Check sheet for the modelled part. Datum: model origin and axes. Units: mm. Face numbers are marked on the shaded views. A direction names the side the tool comes from. Give positions to 0.01 mm unless a question says otherwise; leave off trailing zeros. Order: outer loops, then holes, each group sorted by start corner. A loop starts at its lowest first (then second) coordinate and runs counter-clockwise, first axis right, second up. Notation, with made-up numbers: (65, 25.5) -> (95, 25.5) arc R21 ccw to (95, 50.5) -> close; hole circle Ø7 at (22.25, 71.5). An arc over 180 degrees is marked (long way). One line per question, with ' | ' between items.
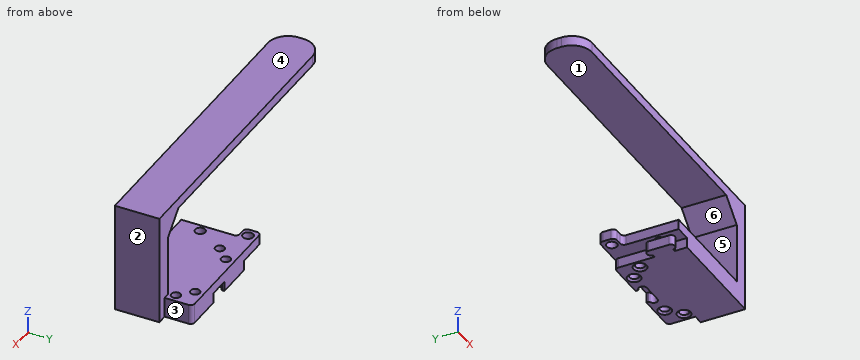
Autodesk Inventor part; units mm, degrees
ref_plane "YZ Plane" through (0, 0, 0) normal (1, 0, 0) x (0, 1, 0)
ref_plane "XZ Plane" through (0, 0, 0) normal (0, 1, 0) x (-1, 0, 0)
ref_plane "XY Plane" through (0, 0, 0) normal (0, 0, 1) x (1, 0, 0)
ref_plane "Arbeitsebene1" through (0, 0, 0) normal (0, 0, 1) x (1, 0, 0)
sketch "Skizze1" plane through (0, 0, 0) normal (0, 0, 1) x (1, 0, 0)
  circle A0 centre (-6.0705, 15.2895) radius 3.5
  circle A1 centre (15.2895, -6.0705) radius 3.5
  line L0 (30.5395, 32.5395) -> (0.0395, 32.5395)
  arc A2 (32.5395, 30.5395) -> (30.5395, 32.5395) centre (30.5395, 30.5395) ccw
  line L1 (32.5395, 30.5395) -> (32.5395, 0.0395)
  arc A3 (30.5395, -1.9605) -> (32.5395, 0.0395) centre (30.5395, 0.0395) ccw
  line L2 (0.0395, -1.9605) -> (30.5395, -1.9605)
  arc A4 (-1.9605, 0.0395) -> (0.0395, -1.9605) centre (0.0395, 0.0395) ccw
  line L3 (-1.9605, 0.0395) -> (-1.9605, 30.5395)
  arc A5 (0.0395, 32.5395) -> (-1.9605, 30.5395) centre (0.0395, 30.5395) ccw
  circle A6 centre (-4.7105, -4.7105) radius 2.45
  circle A7 centre (0.7895, -5.5105) radius 2.3
  circle A8 centre (-5.5105, 0.7895) radius 2.3
  circle A9 centre (-5.5105, 29.7895) radius 2.3
  circle A10 centre (0.7895, 36.0895) radius 2.3
  circle A11 centre (-4.7105, 35.2895) radius 2.45
  circle A12 centre (36.0895, 0.7895) radius 2.3
  circle A13 centre (29.7895, -5.5105) radius 2.3
  circle A14 centre (35.2895, -4.7105) radius 2.45
  circle A15 centre (36.0895, 29.7895) radius 2.3
  circle A16 centre (29.7895, 36.0895) radius 2.3
  circle A17 centre (35.2895, 35.2895) radius 2.45
  line L4 (20.4019, 40.2895) -> (20.4019, 39.1582)
  arc A18 (20.4019, 39.1582) -> (20.6778, 38.7524) centre (20.7437, 39.0939) ccw
  arc A19 (20.2895, 34.6895) -> (20.6778, 38.7524) centre (20.2895, 36.7395) ccw
  line L5 (20.2895, 34.6895) -> (10.1895, 34.6895)
  arc A20 (9.8548, 38.762) -> (10.1895, 34.6895) centre (10.1895, 36.7395) ccw
  arc A21 (9.8548, 38.762) -> (10.1895, 39.1567) centre (9.7895, 39.1567) ccw
  line L6 (10.1895, 39.1567) -> (10.1895, 40.2895)
  line L7 (10.1895, 40.2895) -> (-7.7105, 40.2895)
  arc A22 (-7.7105, 40.2895) -> (-9.7105, 38.2895) centre (-7.7105, 38.2895) ccw
  line L8 (-9.7105, 20.2895) -> (-9.7105, 38.2895)
  line L9 (-10.8433, 20.2895) -> (-9.7105, 20.2895)
  arc A23 (-11.3366, 20.7079) -> (-10.8433, 20.2895) centre (-10.8433, 20.7895) ccw
  arc A24 (-11.3366, 20.7079) -> (-15.2105, 20.3895) centre (-13.2605, 20.3895) ccw
  line L10 (-15.2105, 10.2895) -> (-15.2105, 20.3895)
  arc A25 (-15.2105, 10.2895) -> (-11.3515, 9.8916) centre (-13.2605, 10.2895) ccw
  arc A26 (-10.862, 10.2895) -> (-11.3515, 9.8916) centre (-10.862, 9.7895) ccw
  line L11 (-9.7105, 10.2895) -> (-10.862, 10.2895)
  line L12 (-9.7105, -7.7105) -> (-9.7105, 10.2895)
  arc A27 (-9.7105, -7.7105) -> (-7.7105, -9.7105) centre (-7.7105, -7.7105) ccw
  line L13 (-7.7105, -9.7105) -> (10.2895, -9.7105)
  line L14 (10.2895, -10.8433) -> (10.2895, -9.7105)
  arc A28 (9.8712, -11.3366) -> (10.2895, -10.8433) centre (9.7895, -10.8433) ccw
  arc A29 (9.8712, -11.3366) -> (10.1895, -15.2105) centre (10.1895, -13.2605) ccw
  line L15 (20.2895, -15.2105) -> (10.1895, -15.2105)
  arc A30 (20.2895, -15.2105) -> (20.6875, -11.3515) centre (20.2895, -13.2605) ccw
  arc A31 (20.2895, -10.862) -> (20.6875, -11.3515) centre (20.7895, -10.862) ccw
  line L16 (20.2895, -9.7105) -> (20.2895, -10.862)
  line L17 (20.2895, -9.7105) -> (38.2895, -9.7105)
  arc A32 (38.2895, -9.7105) -> (40.2895, -7.7105) centre (38.2895, -7.7105) ccw
  line L18 (40.2895, 10.1772) -> (40.2895, -7.7105)
  line L19 (40.2895, 10.1772) -> (39.1582, 10.1772)
  arc A33 (39.1582, 10.1772) -> (38.7524, 9.9013) centre (39.0939, 9.8354) ccw
  arc A34 (34.6895, 10.2895) -> (38.7524, 9.9013) centre (36.7395, 10.2895) ccw
  line L20 (34.6895, 10.2895) -> (34.6895, 20.3895)
  arc A35 (38.762, 20.7242) -> (34.6895, 20.3895) centre (36.7395, 20.3895) ccw
  arc A36 (38.762, 20.7242) -> (39.1567, 20.3895) centre (39.1567, 20.7895) ccw
  line L21 (39.1567, 20.3895) -> (40.2895, 20.3895)
  line L22 (40.2895, 38.2895) -> (40.2895, 20.3895)
  arc A37 (40.2895, 38.2895) -> (38.2895, 40.2895) centre (38.2895, 38.2895) ccw
  line L23 (38.2895, 40.2895) -> (20.4019, 40.2895)
  line L24 (40.2895, 26.3895) -> (45.2895, 26.3895)
  line L25 (45.2895, 26.3895) -> (45.2895, 4.1772)
  line L26 (45.2895, 4.1772) -> (40.2895, 4.1772)
  line L27 (40.2895, 4.1772) -> (40.2895, 26.3895)
  point P0 (0, 0)
  dimension "d0" = 5
  dimension "d2" = 6
  dimension "d3" = 6
extrude "Extrusion1" add sketch "Skizze1" along normal blind 5 contours A0 | A2 L1 A3 L2 A4 L3 A5 L0 | A6 | A11 | A14 | A17 | L23 A37 L22 L21 A36 A35 L20 A34 A33 L19 L18 A32 L17 L16 A31 A30 L15 A29 A28 L14 L13 A27 L12 L11 A26 A25 L10 A24 A23 L9 L8 A22 L7 L6 A21 A20 L5 A19 A18 L4 | L24 L25 L26 L18 L27 L22 | L27 L19 A33 A34 L20 A35 A36 L21
chamfer "Fase1" distance 1 angle 45 8 edges at (-1.5105, 36.0895, 0) (27.4895, 36.0895, 0) (33.7895, 29.7895, 0) (33.7895, 0.7895, 0) (27.4895, -5.5105, 0) (-1.5105, -5.5105, 0) (-7.8105, 0.7895, 0) (-7.8105, 29.7895, 0)
sketch "Skizze2" plane through (0, 0, 5) normal (0, 0, 1) x (1, 0, 0)
  line L0 (40.2895, 4.1772) -> (45.2895, 4.1772)
  line L1 (45.2895, 26.3895) -> (40.2895, 26.3895)
  line L2 (45.2895, 4.1772) -> (37.2895, 4.1772)
  line L3 (37.2895, 4.1772) -> (37.2895, 26.3895)
  line L4 (37.2895, 26.3895) -> (45.2895, 26.3895)
  line L5 (45.2895, 26.3895) -> (45.2895, 4.1772)
  point P0 (0, 0)
  point P1 (45.2895, 26.3895)
  point P2 (40.2895, 4.1772)
  dimension "d9" = 8
extrude "Extrusion2" add sketch "Skizze2" along normal blind 45
sketch "Skizze3" plane through (0, 0, 50) normal (0, 0, 1) x (1, 0, 0)
  line L0 (45.2895, 26.3895) -> (37.2895, 26.3895)
  line L1 (37.2895, 26.3895) -> (37.2895, 4.1772)
  line L2 (37.2895, 4.1772) -> (45.2895, 4.1772)
  line L3 (45.2895, 4.1772) -> (45.2895, 26.3895)
  line L4 (45.2895, 26.3895) -> (37.2895, 26.3895)
  line L5 (37.2895, 26.3895) -> (-109.7105, 26.3895)
  line L6 (-109.7105, 26.3895) -> (-109.7105, 4.1772)
  line L7 (-109.7105, 4.1772) -> (37.2895, 4.1772)
  line L8 (37.2895, 4.1772) -> (37.2895, 26.3895)
  circle A0 centre (36.0895, 29.7895) radius 2.3
  circle A1 centre (29.7895, -5.5105) radius 2.3
  circle A2 centre (0.7895, 36.0895) radius 2.3
  circle A3 centre (-5.5105, 29.7895) radius 2.3
  circle A4 centre (-5.5105, 0.7895) radius 2.3
  circle A5 centre (0.7895, -5.5105) radius 2.3
  circle A6 centre (15.2895, -6.0705) radius 3.5
  circle A7 centre (36.0895, 0.7895) radius 2.3
  circle A8 centre (29.7895, 36.0895) radius 2.3
  arc A9 (40.2895, 38.2895) -> (38.2895, 40.2895) centre (38.2895, 38.2895) ccw
  line L9 (38.2895, 40.2895) -> (20.4019, 40.2895)
  line L10 (20.4019, 40.2895) -> (20.4019, 39.1582)
  arc A10 (20.4019, 39.1582) -> (20.6778, 38.7524) centre (20.7437, 39.0939) ccw
  arc A11 (20.2895, 34.6895) -> (20.6778, 38.7524) centre (20.2895, 36.7395) ccw
  line L11 (20.2895, 34.6895) -> (10.1895, 34.6895)
  arc A12 (9.8548, 38.762) -> (10.1895, 34.6895) centre (10.1895, 36.7395) ccw
  arc A13 (9.8548, 38.762) -> (10.1895, 39.1567) centre (9.7895, 39.1567) ccw
  line L12 (10.1895, 39.1567) -> (10.1895, 40.2895)
  line L13 (10.1895, 40.2895) -> (-7.7105, 40.2895)
  arc A14 (-7.7105, 40.2895) -> (-9.7105, 38.2895) centre (-7.7105, 38.2895) ccw
  line L14 (-9.7105, 38.2895) -> (-9.7105, 20.2895)
  line L15 (-9.7105, 20.2895) -> (-10.8433, 20.2895)
  arc A15 (-11.3366, 20.7079) -> (-10.8433, 20.2895) centre (-10.8433, 20.7895) ccw
  arc A16 (-11.3366, 20.7079) -> (-15.2105, 20.3895) centre (-13.2605, 20.3895) ccw
  line L16 (-15.2105, 20.3895) -> (-15.2105, 10.2895)
  arc A17 (-15.2105, 10.2895) -> (-11.3515, 9.8916) centre (-13.2605, 10.2895) ccw
  arc A18 (-10.862, 10.2895) -> (-11.3515, 9.8916) centre (-10.862, 9.7895) ccw
  line L17 (-10.862, 10.2895) -> (-9.7105, 10.2895)
  line L18 (-9.7105, 10.2895) -> (-9.7105, -7.7105)
  arc A19 (-9.7105, -7.7105) -> (-7.7105, -9.7105) centre (-7.7105, -7.7105) ccw
  line L19 (-7.7105, -9.7105) -> (10.2895, -9.7105)
  line L20 (10.2895, -9.7105) -> (10.2895, -10.8433)
  arc A20 (9.8712, -11.3366) -> (10.2895, -10.8433) centre (9.7895, -10.8433) ccw
  arc A21 (9.8712, -11.3366) -> (10.1895, -15.2105) centre (10.1895, -13.2605) ccw
  line L21 (10.1895, -15.2105) -> (20.2895, -15.2105)
  arc A22 (20.2895, -15.2105) -> (20.6875, -11.3515) centre (20.2895, -13.2605) ccw
  arc A23 (20.2895, -10.862) -> (20.6875, -11.3515) centre (20.7895, -10.862) ccw
  line L22 (20.2895, -10.862) -> (20.2895, -9.7105)
  line L23 (20.2895, -9.7105) -> (38.2895, -9.7105)
  arc A24 (38.2895, -9.7105) -> (40.2895, -7.7105) centre (38.2895, -7.7105) ccw
  line L24 (40.2895, -7.7105) -> (40.2895, 4.1772)
  line L25 (37.2895, 4.1772) -> (37.2895, 26.3895)
  line L26 (40.2895, 26.3895) -> (40.2895, 38.2895)
  line L27 (37.2895, 26.3895) -> (40.2895, 26.3895)
  line L28 (40.2895, 4.1772) -> (37.2895, 4.1772)
  point P0 (0, 0)
  dimension "d24" = 100
extrude "Extrusion3" add sketch "Skizze3" along normal blind 5 contours L3 L2 L1 L0 | L1 L7 L18 L17 A18 A17 L16 A16 A15 L15 L14 L5 | L14 L15 A15 A16 L16 A17 A18 L17 L18 L7 L6 L5
chamfer "Fase2" distance 10 angle 45 1 edges at (37.2895, 15.2834, 50)
sketch "Skizze5" plane through (0, 0, 5) normal (0, 0, 1) x (1, 0, 0)
  line L0 (-109.7105, 4.1772) -> (45.2895, 4.1772)
  line L1 (45.2895, 4.1772) -> (45.2895, 26.3895)
  line L2 (45.2895, 26.3895) -> (-109.7105, 26.3895)
  line L3 (-109.7105, 26.3895) -> (-109.7105, 4.1772)
  line L4 (-109.7105, 4.1772) -> (45.2895, 4.1772)
  line L5 (-38.4596, 4.1772) -> (42.3638, 4.1772)
  line L6 (42.3638, 4.1772) -> (42.3638, -19.3333)
  line L7 (42.3638, -19.3333) -> (-38.4596, -19.3333)
  line L8 (-38.4596, -19.3333) -> (-38.4596, 4.1772)
  point P0 (0, 0)
  point P1 (-38.4596, 4.1772)
  point P2 (-38.4596, 4.1772)
extrude "Extrusion5" cut sketch "Skizze5" against normal blind 10 contours L0 L6 L7 L8
fillet "Rundung1" radius 10 2 edges at (-109.7105, 4.1772, 52.5) (-109.7105, 26.3895, 52.5)
sketch "Skizze6" plane through (0, 0, 5) normal (0, 0, 1) x (1, 0, 0)
  circle A0 centre (36.0895, 29.7895) radius 2.3
  circle A1 centre (0.7895, 36.0895) radius 2.3
  circle A2 centre (-5.5105, 29.7895) radius 2.3
  circle A3 centre (29.7895, 36.0895) radius 2.3
  line L0 (-9.7105, 4.1772) -> (37.2895, 4.1772)
  line L1 (37.2895, 26.3895) -> (40.2895, 26.3895)
  line L2 (40.2895, 26.3895) -> (40.2895, 38.2895)
  arc A4 (40.2895, 38.2895) -> (38.2895, 40.2895) centre (38.2895, 38.2895) ccw
  line L3 (38.2895, 40.2895) -> (20.4019, 40.2895)
  line L4 (20.4019, 40.2895) -> (20.4019, 39.1582)
  arc A5 (20.4019, 39.1582) -> (20.6778, 38.7524) centre (20.7437, 39.0939) ccw
  arc A6 (20.2895, 34.6895) -> (20.6778, 38.7524) centre (20.2895, 36.7395) ccw
  line L5 (20.2895, 34.6895) -> (10.1895, 34.6895)
  arc A7 (9.8548, 38.762) -> (10.1895, 34.6895) centre (10.1895, 36.7395) ccw
  arc A8 (9.8548, 38.762) -> (10.1895, 39.1567) centre (9.7895, 39.1567) ccw
  line L6 (10.1895, 39.1567) -> (10.1895, 40.2895)
  line L7 (10.1895, 40.2895) -> (-7.7105, 40.2895)
  arc A9 (-7.7105, 40.2895) -> (-9.7105, 38.2895) centre (-7.7105, 38.2895) ccw
  line L8 (-9.7105, 38.2895) -> (-9.7105, 20.2895)
  line L9 (-9.7105, 20.2895) -> (-10.8433, 20.2895)
  arc A10 (-11.3366, 20.7079) -> (-10.8433, 20.2895) centre (-10.8433, 20.7895) ccw
  arc A11 (-11.3366, 20.7079) -> (-15.2105, 20.3895) centre (-13.2605, 20.3895) ccw
  line L10 (-15.2105, 20.3895) -> (-15.2105, 10.2895)
  arc A12 (-15.2105, 10.2895) -> (-11.3515, 9.8916) centre (-13.2605, 10.2895) ccw
  arc A13 (-10.862, 10.2895) -> (-11.3515, 9.8916) centre (-10.862, 9.7895) ccw
  line L11 (-10.862, 10.2895) -> (-9.7105, 10.2895)
  line L12 (-9.7105, 10.2895) -> (-9.7105, 4.1772)
  circle A14 centre (-20.2105, 36.0895) radius 2.6
  line L13 (20.4019, 40.2895) -> (10.1895, 40.2895)
  line L14 (-9.7105, 40.2895) -> (-17.6105, 40.2895)
  line L15 (-17.6105, 30.3395) -> (-17.6105, 4.1772)
  line L16 (-17.6105, 4.1772) -> (-9.7105, 4.1772)
  line L17 (-9.7105, 4.1772) -> (-9.7105, 40.2895)
  line L18 (-17.6105, 40.2895) -> (-22.6105, 40.2895)
  line L19 (-24.6105, 38.2895) -> (-24.6105, 34.3395)
  line L20 (-22.6105, 32.3395) -> (-19.6105, 32.3395)
  line L21 (-17.6105, 32.3395) -> (-17.6105, 40.2895)
  circle A15 centre (-14.7105, 35.2895) radius 2.425
  circle A16 centre (-13.9105, 29.7895) radius 2.6
  line L22 (27.2895, 4.1772) -> (37.2895, 4.1772)
  line L23 (37.2895, 4.1772) -> (37.2895, 26.3895)
  line L24 (37.2895, 26.3895) -> (27.2895, 26.3895)
  line L25 (27.2895, 26.3895) -> (27.2895, 4.1772)
  circle A17 centre (-13.7105, 15.6895) radius 2.5
  line L26 (37.2895, 4.1772) -> (37.2895, 26.3895)
  line L27 (-9.7105, 40.2895) -> (-7.7105, 40.2895)
  arc A18 (-22.6105, 40.2895) -> (-24.6105, 38.2895) centre (-22.6105, 38.2895) ccw
  arc A19 (-24.6105, 34.3395) -> (-22.6105, 32.3395) centre (-22.6105, 34.3395) ccw
  arc A20 (-17.6105, 30.3395) -> (-19.6105, 32.3395) centre (-19.6105, 30.3395) ccw
  point P0 (0, 0)
  point P1 (-24.6105, 32.3395)
  point P2 (-24.6105, 40.2895)
  point P3 (-17.6105, 32.3395)
  dimension "d25" = 7
  dimension "d28" = 2
extrude "Extrusion6" add sketch "Skizze6" along normal blind 5 contours L12 L17 L8 A9 L7 L6 A8 A7 L5 A6 A5 L4 L3 A4 L2 L1 L24 L25 L0 | L16 L15 A20 L20 A19 L19 A18 L18 L14 L17 L8 L9 A10 A11 L10 A17 A12 A13 L11 L12 | L25 L24 L23 L0 | L11 A13 A12 L10 A17 A11 A10 L9 L17 | L17 L27 A9 | L13 L4 A5 A6 L5 A7 A8 L6 | A15 | A16
properties part number "40_Cube_XY_Table_Illumination_Arm"
Q1. Section check C-C (x = 0). Count the separate pieces of the cut face and the enclosed holes in it, and give its area (3 significant figures).
Result sheet:
separate pieces: 3 | enclosed holes: 0 | area: 428 mm2
Q2. Section check B-B (z = 24). Enter the section's corners in (x, y), and give its area (3 significant figures).
Result sheet:
outline: (37.29, 4.18) -> (45.29, 4.18) -> (45.29, 26.39) -> (37.29, 26.39) -> close | area: 178 mm2
Q3. Mould release check, pull along Z, two halves, no side actions. Record for the marked faces 3, 4, 5 and 6: pulls with the +Z half, pulls with the -Z half, needs draft (parallel to the pull), parting line crosses it, or undercut.
Result sheet:
face 3: needs draft | face 4: pulls with the +Z half | face 5: undercut | face 6: undercut
Q4. Thickness scan on line 1 (Z direction, x = 20.5, y = 8.5); line 2 (Z direction, x = -83, y = 16.5); line 3 (X direction, y = 22, z = 30). Record the ranges inside material, lowest first.
Result sheet:
line 1: z = 0 to 10, 50 to 55 | line 2: z = 50 to 55 | line 3: x = 37.29 to 45.29
Q5. Depth check by flat-ended pin: pin 1 Ø6 at (x, y) = (0.79, 36.09) entering from -Z; pin 2 Ø4 at (x, y) = (-5.51, 29.79) entering from +Z; pin 3 Ø1.5 at (y, z) = (6, 1.5) entering from -X; pin 4 Ø3 at (y, z) = (23, 33.5) entering from -X. Enter the tip coordinate at first touch or a pass-through.
Result sheet:
pin 1: stops at z = 0.3 | pin 2: passes through | pin 3: stops at x = -9.71 | pin 4: stops at x = 37.29
Q6. Access from +Z, -Z, +X, -X, +Y, -Y to the whole of each face (thin tool, end or side, straight path). Record for the marked faces 1 and 2.
Result sheet:
face 1: -X, +Y, -Y | face 2: +Z, -Z, +X, +Y, -Y
Q7. Section check A-A (x = -54). Enter the section's corners in (y, z), and give its area (3 significant figures).
Result sheet:
outline: (4.18, 50) -> (26.39, 50) -> (26.39, 55) -> (4.18, 55) -> close | area: 111 mm2
